Work out the finished part from the listing and answer in its coordinate system (mm). A direction names the side the tool comes from. Give positions to 0.01 mm unless a question says otherwise; leave off trailing zeros. One line per item, written item: value.
from build123d import *

# Parameters (mm, degrees)
SKETCH_1_R      = 2.5
EXTRUDE_1_DEPTH = 350
FILLET_1_R      = 2


with BuildPart() as part:
    # 草图1 → 凸台-拉伸1 (new body)
    with BuildSketch(Plane.XY):
        Polygon((-3.151471863, 4), (3.151471863, 4), (5.45, 6.298528137), (5.45, 8.2), (3.1, 8.2), (3.1, 9.1), (3.6, 9.1), (3.6, 10), (10, 10), (10, 3.6), (9.1, 3.6), (9.1, 3.1), (8.2, 3.1), (8.2, 5.45), (6.298528137, 5.45), (4, 3.151471863), (4, -3.151471863), (6.298528137, -5.45), (8.2, -5.45), (8.2, -3.1), (9.1, -3.1), (9.1, -3.6), (10, -3.6), (10, -10), (3.6, -10), (3.6, -9.1), (3.1, -9.1), (3.1, -8.2), (5.45, -8.2), (5.45, -6.298528137), (3.151471863, -4), (-3.151471863, -4), (-5.45, -6.298528137), (-5.45, -8.2), (-3.1, -8.2), (-3.1, -9.1), (-3.6, -9.1), (-3.6, -10), (-10, -10), (-10, -3.6), (-9.1, -3.6), (-9.1, -3.1), (-8.2, -3.1), (-8.2, -5.45), (-6.298528137, -5.45), (-4, -3.151471863), (-4, 3.151471863), (-6.298528137, 5.45), (-8.2, 5.45), (-8.2, 3.1), (-9.1, 3.1), (-9.1, 3.6), (-10, 3.6), (-10, 10), (-3.6, 10), (-3.6, 9.1), (-3.1, 9.1), (-3.1, 8.2), (-5.45, 8.2), (-5.45, 6.298528137), align=None)
        Circle(SKETCH_1_R, mode=Mode.SUBTRACT)
    extrude(amount=EXTRUDE_1_DEPTH)

    # 圆角1
    fillet_1_edges = [part.edges().sort_by_distance(p)[0] for p in [
        (10, -10, 175),
        (-10, -10, 175),
        (-10, 10, 175),
        (10, 10, 175),
    ]]
    fillet(fillet_1_edges, radius=FILLET_1_R)


solid = part.part
(1) Which of the six approach directions +Z, -Z, +X, -X, +Y, -Y give full straight-line access (tool end or side, diameter ignored) to faces 4 (the flat face through (-2, 2, 350)), 5 (the flat face through (-4, 0, 173))?
Findings:
face 4: +Z, +X, -X, +Y, -Y
face 5: +Z, -Z, -X
(2) Determine the mould class of faces 1 (the flat face through (4, 0, 173)), 2 (the flat face through (-2, 2, 0)), 3 (the flat face through (0, 4, 173)) for opening direction X: pulls with the +X half, pulls with the -X half, needs draft (parallel to the pull), parting line crosses it, or undercut.
Findings:
face 1: pulls with the +X half
face 2: needs draft
face 3: undercut
(3) Find the intervals of material crossed by probe 1 along Y at (x, z) = (0, 85); probe 2 along Y at (x, z) = (6.5, 157.5); probe 3 along X at (y, z) = (0.25, 315.5), in increasing order. Write a range as from..to.
Findings:
probe 1: y = -4..-2.5, 2.5..4
probe 2: y = -10..-5.45, 5.45..10
probe 3: x = -4..-2.49, 2.49..4
(4) Given P1, Ø5, axis at x = 7.5, y = 0.5, coming from the +Z side; P2, Ø1, axis at y = -2.5, z = 234.5, coming from the +X side; P3, Ø0.7, axis at y = -8.5, z = 176.5, coming from the -X side; P4, Ø0.5, axis at y = 8.5, z = 104.5, coming from the +X side, each flat-ended and moving along its own axis, determine where each tip first touches the part or whether it passes through.
Findings:
P1: passes through
P2: stops at x = 4
P3: stops at x = -9.99
P4: stops at x = 9.98
